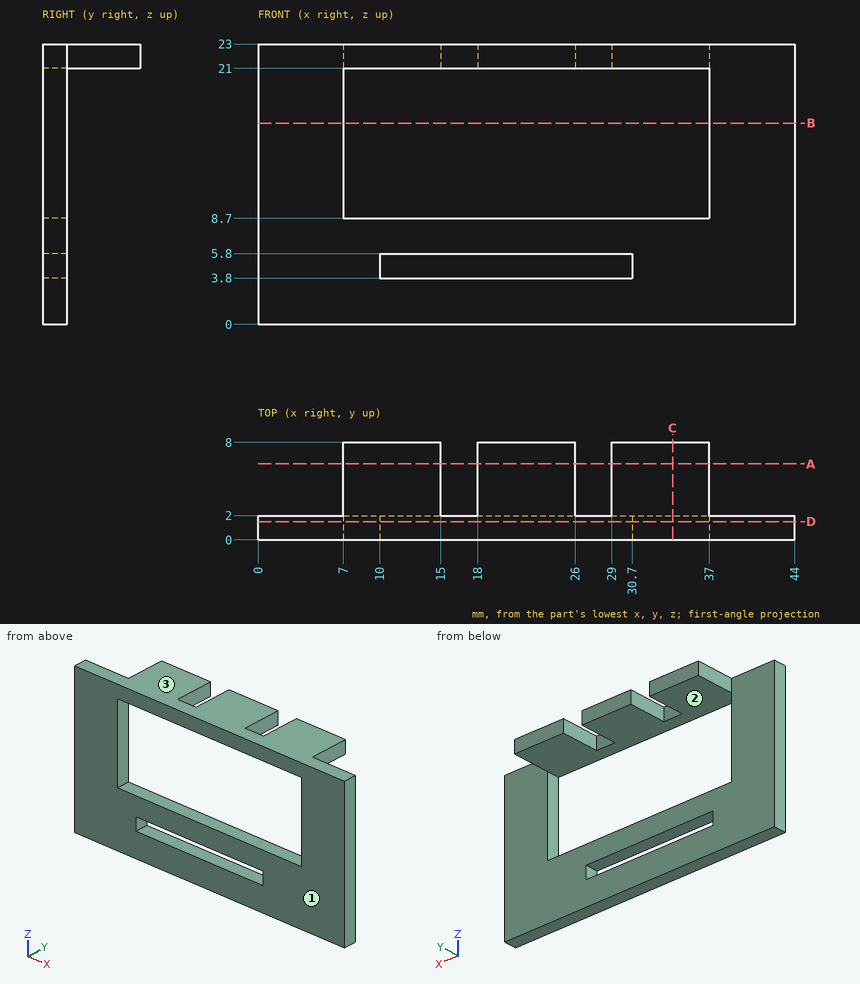
Geometry check sheet. Reference: drawing and pictorial views, mm from the part's lowest x, y, z. Coordinates: 2 decimals unless noted, no trailing zeros. Order: outer loops, then holes, each group sorted by start corner. A loop starts at its lowest first (then second) coordinate and runs counter-clockwise, first axis right, second up. Notation, with made-up numbers: (80.5, -0.75) - (121.5, -0.75) arc R30 cw to (121.5, 27.25) - close; hole circle Ø8 at (54.25, 46.25). An arc over 180 degrees is marked (long way). Answer in a Markdown table with one row per item. Add a question column.
1) Release check for a two-part mould opening along Z. For the marked faces 1, 2 and 3 record: +Z half, -Z half, draft (parallel to the pull), parting line (faces both ways), or undercut.
2) Cross-section at C-C, the plane x = 34. Record the cut outline in (y, z).
3) Cross-section at A-A, the plane y = 6.25. Record the cut outline in (x, z).
4) Cross-section at B-B, the plane z = 16.5. Record the cut outline in (x, y).
5) Gauge pin test, flat ends, axial feed: P1, Ø1.6, axis at y = 5.5, z = 22, coming from the -X side; P2, Ø0.6, axis at y = 1, z = 5, coming from the -X side; P3, Ø2, axis at y = 3.5, z = 22.5, coming from the +X side; P4, Ø7, axis at x = 16, z = 10.5, coming from the +Y side. Record the tip position at first contact, or that the pin passes through.
6) Cross-section at D-D, the plane y = 1.5. Record the cut outline in (x, z).
7) Material ranges on line 1 along X through (y, z) = (7, 22); line 2 along Z through (x, y) = (25, 1.75); line 3 along X through (y, z) = (1.75, 11.75), recorded low to high. Write a range as [from, to].
Check result:
| question | item | result |
|---|---|---|
| 1 | face 1 | draft |
| 1 | face 2 | undercut |
| 1 | face 3 | +Z half |
| 2 | outline | (0, 0) - (2, 0) - (2, 8.7) - (0, 8.7) - close; (0, 21) - (8, 21) - (8, 23) - (0, 23) - close |
| 3 | outline | (7, 21) - (15, 21) - (15, 23) - (7, 23) - close; (18, 21) - (26, 21) - (26, 23) - (18, 23) - close; (29, 21) - (37, 21) - (37, 23) - (29, 23) - close |
| 4 | outline | (0, 0) - (7, 0) - (7, 2) - (0, 2) - close; (37, 0) - (44, 0) - (44, 2) - (37, 2) - close |
| 5 | P1 | stops at x = 7 |
| 5 | P2 | stops at x = 0 |
| 5 | P3 | stops at x = 37 |
| 5 | P4 | stops at y = 2 |
| 6 | outline | (0, 0) - (44, 0) - (44, 23) - (0, 23) - close; hole (7, 8.7) - (37, 8.7) - (37, 21) - (7, 21) - close; hole (10, 3.8) - (30.7, 3.8) - (30.7, 5.8) - (10, 5.8) - close |
| 7 | line 1 | x = [7, 15], [18, 26], [29, 37] |
| 7 | line 2 | z = [0, 3.8], [5.8, 8.7], [21, 23] |
| 7 | line 3 | x = [0, 7], [37, 44] |
